Check sheet for the modelled part. Datum: model origin and axes. Units: mm. Face numbers are marked on the shaded views. A direction names the side the tool comes from. Give positions to 0.01 mm unless a question says otherwise; leave off trailing zeros. Write each loop counter-clockwise with the first axis right and the second up, starting at its lowest first coordinate (ties: lowest second). Pieces come first, ordered by that corner, then holes. Notation, with made-up numbers: (49.25, 3) -> (66.25, 3) arc R29 ccw to (66.25, 28) -> close; hole circle Ø11 at (-36.5, 82.25). An arc over 180 degrees is marked (long way). Answer as a JSON object with one key per item and string values.
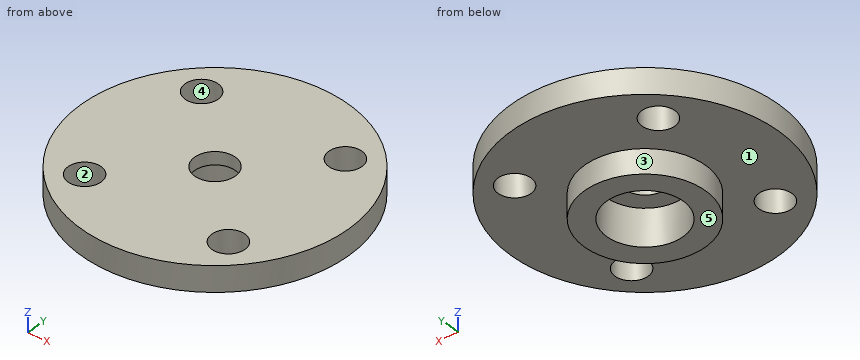
from build123d import *

# Parameters (mm, degrees)
SKETCH_2_R               = 2.6
CUT_EXTRUDE_1_DEPTH      = 4
PATTERN_CIRCULAR_1_COUNT = 4


with BuildPart() as part:
    # Эскиз1 → Повернуть1 (revolve)
    with BuildSketch(Plane(origin=(0, 0, 0), x_dir=(1, 0, 0), z_dir=(0, 1, 0)), mode=Mode.PRIVATE) as revolve_1_sk:
        Polygon((-3.2, 0), (-21, 0), (-21, 4), (-9.5, 4), (-9.5, 7.8), (-6, 7.8), (-6, 2), (-3.2, 2), align=None)
    revolve(revolve_1_sk.sketch.rotate(Axis((0, 0, 0), (0, 0, -1)), 180), axis=Axis((0, 0, 0), (0, 0, -1)))

    # Эскиз2 → Вырез-Вытянуть1 (cut)
    with BuildSketch(Plane.XY):
        with Locations((11.313708499, 11.313708499)):
            Circle(SKETCH_2_R)
    cut_extrude_1 = extrude(amount=-CUT_EXTRUDE_1_DEPTH, mode=Mode.SUBTRACT)

    # Круговой массив1: Вырез-Вытянуть1 ×4 about axis
    pattern_circular_1_axis = Axis((0, 0, 0), (0, 0, 1))
    for i in range(1, PATTERN_CIRCULAR_1_COUNT):
        add(cut_extrude_1.rotate(pattern_circular_1_axis, i * 360 / PATTERN_CIRCULAR_1_COUNT), mode=Mode.SUBTRACT)


solid = part.part
1. Sectioned sample at C-C, the plane x = 13. Enter the section's corners in (y, z).
Determined:
{"outline": "(-16.49, -4) -> (-13.29, -4) -> (-13.29, 0) -> (-16.49, 0) -> close; (-9.33, -4) -> (9.33, -4) -> (9.33, 0) -> (-9.33, 0) -> close; (13.29, -4) -> (16.49, -4) -> (16.49, 0) -> (13.29, 0) -> close"}
2. Go/stop test with flat-tipped pins: P1, Ø4, axis at x = 13.5, z = -2, coming from the -Y side; P2, Ø8.5, axis at x = 11.31, y = -11.31, coming from the -Z side; P3, Ø6, axis at x = -1, y = 1.5, coming from the -Z side. Record where each tip stops, or that it passes through.
Determined:
{"P1": "y = -17.57", "P2": "z = -4", "P3": "z = -2"}
3. Sectioned sample at D-D, the plane y = 10.5. Enter the section's corners in (x, z), plus the area to 3 significant figures.
Determined:
{"outline": "(-18.19, -4) -> (-13.78, -4) -> (-13.78, 0) -> (-18.19, 0) -> close; (-8.84, -4) -> (8.84, -4) -> (8.84, 0) -> (-8.84, 0) -> close; (13.78, -4) -> (18.19, -4) -> (18.19, 0) -> (13.78, 0) -> close", "area": "106 mm^2"}
4. Sectioned sample at A-A, the plane x = 0. Enter the section's corners in (y, z).
Determined:
{"outline": "(-21, -4) -> (-9.5, -4) -> (-9.5, -7.8) -> (-6, -7.8) -> (-6, -2) -> (-3.2, -2) -> (-3.2, 0) -> (-21, 0) -> close; (3.2, -2) -> (6, -2) -> (6, -7.8) -> (9.5, -7.8) -> (9.5, -4) -> (21, -4) -> (21, 0) -> (3.2, 0) -> close"}
5. Mould release check, pull along X, two halves, no side actions. Record for the marked faces 3, 4 and 5: released by +X, released by -X, zero draft, split by the parting line, or undercut.
Determined:
{"face 3": "split by the parting line", "face 4": "undercut", "face 5": "zero draft"}
6. Access from +Z, -Z, +X, -X, +Y, -Y to the whole of each face (thin tool, end or side, straight path). Record for the marked faces 1 and 2.
Determined:
{"face 1": "-Z", "face 2": "+Z, -Z"}
7. Scan lines: L1, parallel to X at y = 12, z = -0.25; L2, parallel to Y at x = 0, z = -1; L3, parallel to Y at x = -9.5, z = -2. Record each from-to range of solid material in increasing order. Write a range as [from, to].
Determined:
{"L1": "[-17.23, -13.82], [-8.81, 8.81], [13.82, 17.23]", "L2": "[-21, -3.2], [3.2, 21]", "L3": "[-18.73, -13.18], [-9.45, 9.45], [13.18, 18.73]"}
